For this review, take the finished solid that the model builds, in its own axes (mm). A direction names the side the tool comes from. Round coordinates to 2 decimals unless told otherwise and drop trailing zeros. Loops run counter-clockwise (first coordinate to the right, second up) from the corner with the lowest first, then second, coordinate; pieces in that order, holes last.
1) Tool access review of faces 1 (the flat face through (-2, -6, -255)), 2 (the conical face through (192.99, -4.85, 197.13)), 3 (the cylindrical face through (191.62, -0.99, -194.47)): name each direction out of +Z, -Z, +X, -X, +Y, -Y from which nothing blocks a thin tool from reaching the whole face with its end or side.
2) Take a section at B-B (z = 143). State the section outline as (x, y) points, then the cut area to 3 significant figures.
3) Take a section at C-C (y = -6.75). State the section outline as (x, z) points.
4) Insertion check: pin 1 (2 mm diameter, centred on y = -8, z = 170, fed in from +X); pin 2 (0.6 mm diameter, centred on y = -1, z = -10, fed in from -X); pin 3 (1.5 mm diameter, centred on y = -6, z = -43, fed in from +X); pin 4 (12 mm diameter, centred on x = -161.5, z = -198, fed in from -Y). Each pin has a flat end and moves straight along its axis. Give the tip position at first contact, or say it passes through.
5) Mouldability with a two-part tool opening along Z and no side actions: class faces 4 (the conical face through (-190.604, -4.848, 196.463)), 5 (the flat face through (-2, -6, 255)), 6 (the flat face through (-221, -12, 20)), 7 (the conical face through (193.654, -4.848, -196.463)) as pulls with the +Z half, pulls with the -Z half, needs draft (parallel to the pull), parting line crosses it, or undercut.
6) Wall thickness on L1, parallel to Z at x = -69, y = -1; L2, parallel to Z at x = -130, y = -6; L3, parallel to X at y = -2.5, z = 69: over which ranges is each line inside the solid? List them lowest first.
7) Take a section at A-A (x = -136). State the section outline as (y, z) points, then the cut area to 3 significant figures.
```python
from build123d import *

# Parameters (mm, degrees)
F0_W        = 500
F0_H        = 510
F1_DEPTH    = 12
F2_SIZE     = 10
F3_T1_DEPTH = 607.9795897113


# Not quite as in the source:
# - a fillet or chamfer that OpenCascade refuses, or shapes differently, is made with other operations: its cross-section is extruded or revolved along the edge and cut away or added


with BuildPart() as f1:
    # F0 (on Front) → F1 (new body)
    with BuildSketch(Plane.XZ):
        with Locations((1.5247634146, 0)):
            Rectangle(F0_W, F0_H)
        with BuildLine():
            ThreePointArc((-199.9752365854, 166.5), (-188.2595078328, 194.7842712475), (-159.9752365854, 206.5))
            Line((-159.9752365854, 206.5), (163.0247634146, 206.5))
            ThreePointArc((163.0247634146, 206.5), (191.3090346621, 194.7842712475), (203.0247634146, 166.5))
            Line((203.0247634146, 166.5), (203.0247634146, -166.5))
            ThreePointArc((203.0247634146, -166.5), (191.3090346621, -194.7842712475), (163.0247634146, -206.5))
            Line((163.0247634146, -206.5), (-159.9752365854, -206.5))
            ThreePointArc((-159.9752365854, -206.5), (-188.2595078328, -194.7842712475), (-199.9752365854, -166.5))
            Line((-199.9752365854, -166.5), (-199.9752365854, 166.5))
        make_face(mode=Mode.SUBTRACT)
    extrude(amount=F1_DEPTH)

    # F2
    f2_edges = [f1.edges().sort_by_distance(p)[0] for p in [
        (1.524763, -12, 206.5),
        (-199.975237, -12, 0),
        (-188.259508, -12, 194.784271),
        (191.309035, -12, 194.784271),
        (203.024763, -12, 0),
        (191.309035, -12, -194.784271),
        (1.524763, -12, -206.5),
        (-188.259508, -12, -194.784271),
    ]]
    chamfer(f2_edges, length=F2_SIZE)

    # F3: fillet of radius 22 on 2 edges, made by hand

    # F3_s2 → F3_t1 (cut)
    with BuildSketch(Plane.XY.offset(-303.9897948557)):
        with BuildLine():
            ThreePointArc((-228.8793186431, -12), (-240.3684439362, -8.7616630393), (-248.4752365854, 0))
            Line((-248.4752365854, 0), (-248.4752365854, -12))
            Line((-248.4752365854, -12), (-228.8793186431, -12))
        make_face()
        with BuildLine():
            ThreePointArc((231.9288454724, -12), (243.4179707654, -8.7616630393), (251.5247634146, 0))
            Line((251.5247634146, 0), (251.5247634146, -12))
            Line((251.5247634146, -12), (231.9288454724, -12))
        make_face()
    extrude(amount=F3_T1_DEPTH, mode=Mode.SUBTRACT)


solid = f1.part
```
Response:
1. face 1: -Z, +X, -X, +Y, -Y
1. face 2: -Y
1. face 3: +Y, -Y
2. outline: (-248.48, 0) arc R22 ccw to (-228.88, -12) - (-209.98, -12) - (-199.98, -2) - (-199.98, 0) - close; (203.02, -2) - (213.02, -12) - (231.93, -12) arc R22 ccw to (251.52, 0) - (203.02, 0) - close
2. area: 930 mm2
3. outline: (-243.14, -255) - (246.19, -255) - (246.19, 255) - (-243.14, 255) - close; hole (-204.73, -166.5) arc R44.75 ccw to (-159.98, -211.25) - (163.02, -211.25) arc R44.75 ccw to (207.77, -166.5) - (207.77, 166.5) arc R44.75 ccw to (163.02, 211.25) - (-159.98, 211.25) arc R44.75 ccw to (-204.73, 166.5) - close
4. pin 1: stops at x = 245.89
4. pin 2: stops at x = -248.1
4. pin 3: stops at x = 247.79
4. pin 4: passes through
5. face 4: undercut
5. face 5: pulls with the +Z half
5. face 6: needs draft
5. face 7: undercut
6. L1: z = -255 to -206.5, 206.5 to 255
6. L2: z = -255 to -210.5, 210.5 to 255
6. L3: x = -246.98 to -200.48, 203.52 to 250.03
7. outline: (-12, -255) - (0, -255) - (0, -206.5) - (-2, -206.5) - (-12, -216.5) - close; (-12, 216.5) - (-2, 206.5) - (0, 206.5) - (0, 255) - (-12, 255) - close
7. area: 1,060 mm2
